```python
from build123d import *

# Parameters (mm, degrees)
ESQUISSE1_R             = 46
ESQUISSE1_R_2           = 38
BOSS_EXTRU_1_DEPTH      = 1.6
ESQUISSE2_R             = 0.9
ENL_V_MAT_EXTRU_1_DEPTH = 1.6
ESQUISSE3_W             = 5
ESQUISSE3_H             = 5
BOSS_EXTRU_2_DEPTH      = 1.8


with BuildPart() as part:
    # Esquisse1 → Boss.-Extru.1 (new body)
    with BuildSketch(Plane(origin=(0, 0, 0), x_dir=(1, 0, 0), z_dir=(0, 1, 0))):
        with Locations(Location((0, 0, 0), (0, 0, 270))):
            Circle(ESQUISSE1_R)
        with Locations(Location((0, 0, 0), (0, 0, 270))):
            Circle(ESQUISSE1_R_2, mode=Mode.SUBTRACT)
    extrude(amount=BOSS_EXTRU_1_DEPTH)

    # Esquisse2 → Enlèv. mat.-Extru.1 (cut)
    with BuildSketch(Plane(origin=(0, 1.6, 0), x_dir=(1, 0, 0), z_dir=(0, 1, 0))):
        with Locations(Location((-4.094938915, 44.411614194, 0), (0, 0, 270))):
            Circle(ESQUISSE2_R)
        with Locations(Location((44.411614194, 4.094938915, 0), (0, 0, 270))):
            Circle(ESQUISSE2_R)
        with Locations(Location((4.094938915, -44.411614194, 0), (0, 0, 270))):
            Circle(ESQUISSE2_R)
        with Locations(Location((-44.411614194, -4.094938915, 0), (0, 0, 270))):
            Circle(ESQUISSE2_R)
    extrude(amount=-ENL_V_MAT_EXTRU_1_DEPTH, mode=Mode.SUBTRACT)

    # Esquisse3 → Boss.-Extru.2 (add)
    with BuildSketch(Plane(origin=(0, 1.6, 0), x_dir=(1, 0, 0), z_dir=(0, 1, 0))):
        with Locations((0, 42.5)):
            Rectangle(ESQUISSE3_W, ESQUISSE3_H)
        Polygon((9.232042464, 44.113709796), (14.061671595, 42.81961457), (12.76757637, 37.989985439), (7.937947238, 39.284080664), align=None)
        Polygon((20.334936491, 40.22114317), (24.665063509, 37.72114317), (22.165063509, 33.391016151), (17.834936491, 35.891016151), align=None)
        Polygon((30.0520382, 33.587572106), (33.587572106, 30.0520382), (30.0520382, 26.516504294), (26.516504294, 30.0520382), align=None)
        Polygon((37.72114317, 24.665063509), (40.22114317, 20.334936491), (35.891016151, 17.834936491), (33.391016151, 22.165063509), align=None)
        Polygon((42.81961457, 14.061671595), (44.113709796, 9.232042464), (39.284080664, 7.937947238), (37.989985439, 12.76757637), align=None)
        with Locations((42.5, 0)):
            Rectangle(ESQUISSE3_W, ESQUISSE3_H)
        Polygon((44.113709796, -9.232042464), (42.81961457, -14.061671595), (37.989985439, -12.76757637), (39.284080664, -7.937947238), align=None)
        Polygon((40.22114317, -20.334936491), (37.72114317, -24.665063509), (33.391016151, -22.165063509), (35.891016151, -17.834936491), align=None)
        Polygon((33.587572106, -30.0520382), (30.0520382, -33.587572106), (26.516504294, -30.0520382), (30.0520382, -26.516504294), align=None)
        Polygon((24.665063509, -37.72114317), (20.334936491, -40.22114317), (17.834936491, -35.891016151), (22.165063509, -33.391016151), align=None)
        Polygon((14.061671595, -42.81961457), (9.232042464, -44.113709796), (7.937947238, -39.284080664), (12.76757637, -37.989985439), align=None)
        with Locations((0, -42.5)):
            Rectangle(ESQUISSE3_W, ESQUISSE3_H)
        Polygon((-9.232042464, -44.113709796), (-14.061671595, -42.81961457), (-12.76757637, -37.989985439), (-7.937947238, -39.284080664), align=None)
        Polygon((-20.334936491, -40.22114317), (-24.665063509, -37.72114317), (-22.165063509, -33.391016151), (-17.834936491, -35.891016151), align=None)
        Polygon((-30.0520382, -33.587572106), (-33.587572106, -30.0520382), (-30.0520382, -26.516504294), (-26.516504294, -30.0520382), align=None)
        Polygon((-37.72114317, -24.665063509), (-40.22114317, -20.334936491), (-35.891016151, -17.834936491), (-33.391016151, -22.165063509), align=None)
        Polygon((-42.81961457, -14.061671595), (-44.113709796, -9.232042464), (-39.284080664, -7.937947238), (-37.989985439, -12.76757637), align=None)
        with Locations((-42.5, 0)):
            Rectangle(ESQUISSE3_W, ESQUISSE3_H)
        Polygon((-44.113709796, 9.232042464), (-42.81961457, 14.061671595), (-37.989985439, 12.76757637), (-39.284080664, 7.937947238), align=None)
        Polygon((-40.22114317, 20.334936491), (-37.72114317, 24.665063509), (-33.391016151, 22.165063509), (-35.891016151, 17.834936491), align=None)
        Polygon((-33.587572106, 30.0520382), (-30.0520382, 33.587572106), (-26.516504294, 30.0520382), (-30.0520382, 26.516504294), align=None)
        Polygon((-24.665063509, 37.72114317), (-20.334936491, 40.22114317), (-17.834936491, 35.891016151), (-22.165063509, 33.391016151), align=None)
        Polygon((-14.061671595, 42.81961457), (-9.232042464, 44.113709796), (-7.937947238, 39.284080664), (-12.76757637, 37.989985439), align=None)
    extrude(amount=BOSS_EXTRU_2_DEPTH)


solid = part.part
```
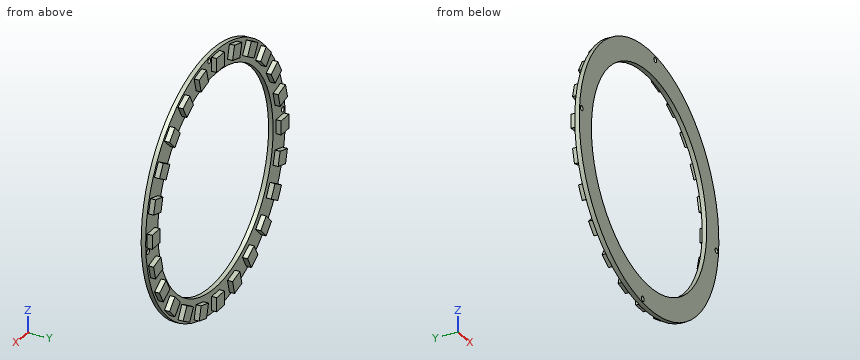
Input: part model. Units: mm. Frame: model coordinates. Coordinates: 2 decimals unless noted, no trailing zeros. Order: outer loops, then holes, each group sorted by start corner. A loop starts at its lowest first (then second) coordinate and runs counter-clockwise, first axis right, second up. Notation, with made-up numbers: (69.25, 79.25) - (93.25, 79.25) arc R30 ccw to (93.25, 117.25) - close; hole circle Ø9 at (42, 51). An arc over 180 degrees is marked (long way). Return JSON: item names as keys, results as strings.
Q1. Cut plane C-C (y = 2.25). State how many separate pieces and enclosed holes the cut face has, then the cut area to 3 significant figures.
The answers:
{"separate pieces": "24", "enclosed holes": "0", "area": "600 mm2"}
Q2. Cut plane A-A (z = 0). Return loops of the section in (x, y).
The answers:
{"outline": "(-46, 0) - (-38, 0) - (-38, 1.6) - (-40, 1.6) - (-40, 3.4) - (-45, 3.4) - (-45, 1.6) - (-46, 1.6) - close; (38, 0) - (46, 0) - (46, 1.6) - (45, 1.6) - (45, 3.4) - (40, 3.4) - (40, 1.6) - (38, 1.6) - close"}
Q3. Cut plane B-B (x = 0). Return loops of the section in (y, z), then the cut area to 3 significant figures.
The answers:
{"outline": "(0, -46) - (1.6, -46) - (1.6, -45) - (3.4, -45) - (3.4, -40) - (1.6, -40) - (1.6, -38) - (0, -38) - close; (0, 38) - (1.6, 38) - (1.6, 40) - (3.4, 40) - (3.4, 45) - (1.6, 45) - (1.6, 46) - (0, 46) - close", "area": "43.6 mm2"}
Q4. Cut plane D-D (z = -16.5). Return loops of the section in (x, y).
The answers:
{"outline": "(-42.94, 0) - (-34.23, 0) - (-34.23, 1.6) - (-42.94, 1.6) - close; (34.23, 0) - (42.94, 0) - (42.94, 1.6) - (34.23, 1.6) - close"}
Q5. Ray query, probe 1 along X at (y, z) = (1.65, 42); probe 2 along Z at (x, y) = (-33, 3.1); probe 3 along X at (y, z) = (1.15, 23.5). Return the intervals inside material, ascending.
The answers:
{"probe 1": "x = -13.84 to -8.67, -2.5 to 2.5, 8.67 to 13.84", "probe 2": "z = -30.64 to -29.46, 29.46 to 30.64", "probe 3": "x = -39.54 to -29.86, 29.86 to 39.54"}
Q6. First-contact query: pin 1 (2 mm diameter, centred on x = 41.5, y = 2, fed in from +Z); pin 2 (8 mm diameter, centred on x = -27, z = 15, fed in from +Y); pin 3 (0.9 mm diameter, centred on y = 2.5, z = -0.5, fed in from -X); pin 4 (0.9 mm diameter, centred on x = -42.5, y = 2.5, fed in from +Z). Flat tips, straight axial feed; report the tip coordinate or a pass-through.
The answers:
{"pin 1": "stops at z = 21.66", "pin 2": "passes through", "pin 3": "stops at x = -45", "pin 4": "stops at z = 14.06"}
